from build123d import *

# Parameters (mm, degrees)
F0_W        = 102.9718667269
F0_H        = 59.044812806
F1_DEPTH    = 72.898
F2_W        = 14.8325152695
F2_H        = 63.3234274574
F2_W_2      = 15.6882368028
F2_H_2      = 63.3234172128
F2_W_3      = 15.1177551597
F2_H_3      = 63.8939035125
F2_W_4      = 36.5108018741
F2_H_4      = 27.9535762966
F2_H_5      = 31.0912323184
F4_DEPTH    = 47.498
F5_T1_DEPTH = 329.8596573187


# Not quite as in the source:
# - a fillet or chamfer that OpenCascade refuses, or shapes differently, is made with other operations: its cross-section is extruded or revolved along the edge and cut away or added


with BuildPart() as f1:
    # F0 (on Front) → F1 (new body)
    with BuildSketch(Plane.XZ):
        with Locations((0.1426190138, -18.5406408273)):
            Rectangle(F0_W, F0_H)
    extrude(amount=-F1_DEPTH)

    # F2 (on face) → F4 (cut)
    with BuildSketch(Plane.XY.offset(10.9817655757)):
        with Locations((-38.7927275151, 36.0829436686)):
            Rectangle(F2_W, F2_H)
        with Locations((-20.1094653457, 36.3681793679)):
            Rectangle(F2_W_2, F2_H_2)
        with Locations((-0.7131015882, 36.3681816962)):
            Rectangle(F2_W_3, F2_H_3)
        with Locations((29.3797855265, 54.6235833317)):
            Rectangle(F2_W_4, F2_H_4)
        with Locations((29.3797855265, 19.9668460991)):
            Rectangle(F2_W_4, F2_H_5)
    extrude(amount=-F4_DEPTH, mode=Mode.SUBTRACT)

    # F5: fillet of radius 45.3775581184 on 1 edges, made by hand

    # F5_s2 → F5_t1 (cut)
    with BuildSketch(Plane.YZ.offset(-164.7872096456)):
        with BuildLine():
            ThreePointArc((27.5204418816, 10.9817655757), (59.6072209408, -2.3090134835), (72.898, -34.3957925427))
            Line((72.898, -34.3957925427), (72.898, 10.9817655757))
            Line((72.898, 10.9817655757), (27.5204418816, 10.9817655757))
        make_face()
    extrude(amount=F5_T1_DEPTH, mode=Mode.SUBTRACT)


solid = f1.part
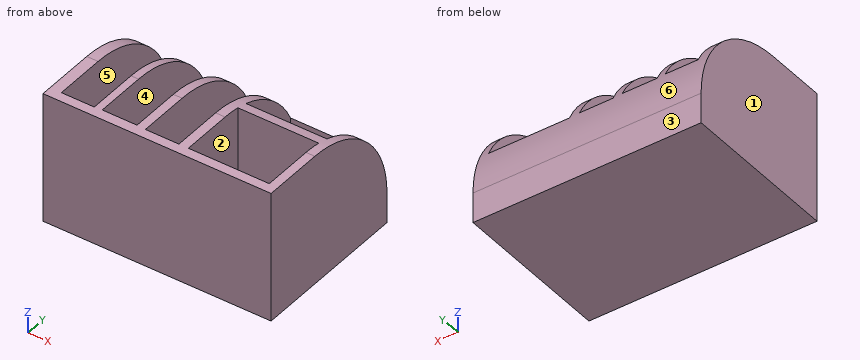
Could you check a few things on this model? Use its own coordinates, in mm. Face numbers are marked on the shaded views. A direction names the side the tool comes from. Coordinates: 2 decimals unless noted, no trailing zeros. Order: outer loops, then holes, each group sorted by start corner. A loop starts at its lowest first (then second) coordinate and runs counter-clockwise, first axis right, second up. Notation, with made-up numbers: (45, -10.75) -> (84, -10.75) arc R31 cw to (84, 17.25) -> close; hole circle Ø4 at (9, -31.75). An arc over 180 degrees is marked (long way). One line per question, with ' | ' between items.
Q1. I'm going to push flat-ended pins straight in: P1, Ø8, axis at x = -17, z = -7.5, coming from the +Y side; P2, Ø6, axis at x = -40, z = -13, coming from the +Y side; P3, Ø12, axis at x = -0.5, y = 24, coming from the +Z side. Where does each tip first touch, or does it pass through?
Return value:
P1: y = 4.71 | P2: y = 69 | P3: z = -36.52
Q2. Imagine slicing it at C-C on z = 3. Please give me the cut outline in (x, y).
Return value:
outline: (-51.34, 0) -> (51.63, 0) -> (51.63, 53.22) -> (47.64, 53.22) -> (47.64, 40.65) -> (11.12, 40.65) -> (11.12, 53.22) -> (6.85, 53.22) -> (6.85, 4.42) -> (-8.27, 4.42) -> (-8.27, 53.22) -> (-12.27, 53.22) -> (-12.27, 4.71) -> (-27.95, 4.71) -> (-27.95, 53.22) -> (-31.38, 53.22) -> (-31.38, 4.42) -> (-46.21, 4.42) -> (-46.21, 53.22) -> (-51.34, 53.22) -> close; hole (11.12, 4.42) -> (47.64, 4.42) -> (47.64, 35.51) -> (11.12, 35.51) -> close
Q3. Imagine slicing it at A-A on x = 40. Please give me the cut outline in (y, z), and give its area (3 significant figures).
Return value:
outline: (0, -48.06) -> (72.9, -48.06) -> (72.9, -34.4) arc R45.38 ccw to (68.6, -15.12) -> (68.6, -36.52) -> (40.65, -36.52) -> (40.65, 9.04) arc R45.38 ccw to (35.51, 10.27) -> (35.51, -36.52) -> (4.42, -36.52) -> (4.42, 10.98) -> (0, 10.98) -> close | area: 1,350 mm²
Q4. If I drill on L1, parallel to X at y = 60, z = -6; L2, parallel to X at y = 36, z = 7; L3, parallel to Y at x = 13, z = -11, over which ranges is the centre line in solid material (lowest first)?
Return value:
L1: -51.34 to -46.21, -31.38 to -27.95, -12.27 to -8.27, 6.85 to 11.12, 47.64 to 51.63 | L2: -51.34 to -46.21, -31.38 to -27.95, -12.27 to -8.27, 6.85 to 51.63 | L3: 0 to 4.42, 35.51 to 40.65
Q5. Thinking about a two-plate mould opening in Y: for the marked faces 1, 2, 3 and 4, which applies, pulls with the +Y half, pulls with the -Y half, needs draft (parallel to the pull), parting line crosses it, or undercut?
Return value:
face 1: needs draft | face 2: undercut | face 3: pulls with the +Y half | face 4: undercut
Q6. On a 3-axis mill with a long thin cutter (end or side, diameter ignored), from which of +Z, -Z, +X, -X, +Y, -Y can I reach the whole of each face in a straight line? I mean the marked faces 5 and 6. Say none if no direction works.
Return value:
face 5: +Z | face 6: +Z, +X, -X, +Y
Q7. Imagine slicing it at B-B on z = -25. Please give me the cut outline in (x, y), and give its area (3 significant figures).
Return value:
outline: (-51.34, 0) -> (51.63, 0) -> (51.63, 71.91) -> (-51.34, 71.91) -> close; hole (-46.21, 4.42) -> (-31.38, 4.42) -> (-31.38, 67.74) -> (-46.21, 67.74) -> close; hole (-27.95, 4.71) -> (-12.27, 4.71) -> (-12.27, 68.03) -> (-27.95, 68.03) -> close; hole (-8.27, 4.42) -> (6.85, 4.42) -> (6.85, 68.32) -> (-8.27, 68.32) -> close; hole (11.12, 4.42) -> (47.64, 4.42) -> (47.64, 35.51) -> (11.12, 35.51) -> close; hole (11.12, 40.65) -> (47.64, 40.65) -> (47.64, 68.6) -> (11.12, 68.6) -> close | area: 2,350 mm²
Q8. Imagine slicing it at D-D on y = 19.5. Please give me the cut outline in (x, z).
Return value:
outline: (-51.34, -48.06) -> (51.63, -48.06) -> (51.63, 10.98) -> (47.64, 10.98) -> (47.64, -36.52) -> (11.12, -36.52) -> (11.12, 10.98) -> (6.85, 10.98) -> (6.85, -36.52) -> (-8.27, -36.52) -> (-8.27, 10.98) -> (-12.27, 10.98) -> (-12.27, -36.52) -> (-27.95, -36.52) -> (-27.95, 10.98) -> (-31.38, 10.98) -> (-31.38, -36.52) -> (-46.21, -36.52) -> (-46.21, 10.98) -> (-51.34, 10.98) -> close
